from build123d import *

# Parameters (mm, degrees)
CROQUIS1_R                 = 1.35255
CROQUIS1_R_2               = 1.778
SALIENTE_EXTRUIR1_DEPTH    = 3.175
CROQUIS5_R                 = 2.55
CORTAR_EXTRUIR1_DEPTH      = 53.649355209
CORTAR_EXTRUIR2_DEPTH      = 53.649355209
CORTAR_EXTRUIR2_DEPTH_BACK = 53.649355209
CROQUIS10_R                = 2.078
CROQUIS10_R_2              = 1.65255
CROQUIS10_R_3              = 2.85
CORTAR_EXTRUIR3_DEPTH      = 53.649355209


with BuildPart() as part:
    # Croquis1 → Saliente-Extruir1 (new body)
    with BuildSketch(Plane.XZ):
        with BuildLine():
            Line((-6.02234, -19.2405), (-6.02234, -20.828))
            ThreePointArc((-6.02234, -20.828), (-5.836352806, -21.277012806), (-5.38734, -21.463))
            Line((-5.38734, -21.463), (0.96266, -21.463))
            ThreePointArc((0.96266, -21.463), (1.411672806, -21.277012806), (1.59766, -20.828))
            Line((1.59766, -20.828), (1.59766, -19.2405))
            ThreePointArc((1.59766, -19.2405), (2.062627985, -18.117967985), (3.18516, -17.653))
            Line((3.18516, -17.653), (36.43122, -17.653))
            ThreePointArc((36.43122, -17.653), (41.454190356, -15.572417555), (43.534772801, -10.549447199))
            Line((43.534772801, -10.549447199), (43.534772801, 10.549447199))
            ThreePointArc((43.534772801, 10.549447199), (41.454190356, 15.572417555), (36.43122, 17.653))
            Line((36.43122, 17.653), (3.18516, 17.653))
            ThreePointArc((3.18516, 17.653), (2.062627985, 18.117967985), (1.59766, 19.2405))
            Line((1.59766, 19.2405), (1.59766, 20.828))
            ThreePointArc((1.59766, 20.828), (1.411672806, 21.277012806), (0.96266, 21.463))
            Line((0.96266, 21.463), (-5.38734, 21.463))
            ThreePointArc((-5.38734, 21.463), (-5.836352806, 21.277012806), (-6.02234, 20.828))
            Line((-6.02234, 20.828), (-6.02234, 19.2405))
            ThreePointArc((-6.02234, 19.2405), (-6.487307985, 18.117967985), (-7.60984, 17.653))
            Line((-7.60984, 17.653), (-23.755604, 17.653))
            ThreePointArc((-23.755604, 17.653), (-24.878136015, 18.117967985), (-25.343104, 19.2405))
            Line((-25.343104, 19.2405), (-25.343104, 20.828))
            ThreePointArc((-25.343104, 20.828), (-25.529091194, 21.277012806), (-25.978104, 21.463))
            Line((-25.978104, 21.463), (-32.328104, 21.463))
            ThreePointArc((-32.328104, 21.463), (-32.777116806, 21.277012806), (-32.963104, 20.828))
            Line((-32.963104, 20.828), (-32.963104, 19.2405))
            ThreePointArc((-32.963104, 19.2405), (-33.428071985, 18.117967985), (-34.550604, 17.653))
            Line((-34.550604, 17.653), (-36.43122, 17.653))
            ThreePointArc((-36.43122, 17.653), (-44.591052878, 14.273086555), (-47.970966323, 6.113253677))
            Line((-47.970966323, 6.113253677), (-47.970966323, -6.113253677))
            ThreePointArc((-47.970966323, -6.113253677), (-44.591052878, -14.273086555), (-36.43122, -17.653))
            Line((-36.43122, -17.653), (-34.550604, -17.653))
            ThreePointArc((-34.550604, -17.653), (-33.428071985, -18.117967985), (-32.963104, -19.2405))
            Line((-32.963104, -19.2405), (-32.963104, -20.828))
            ThreePointArc((-32.963104, -20.828), (-32.777116806, -21.277012806), (-32.328104, -21.463))
            Line((-32.328104, -21.463), (-25.978104, -21.463))
            ThreePointArc((-25.978104, -21.463), (-25.529091194, -21.277012806), (-25.343104, -20.828))
            Line((-25.343104, -20.828), (-25.343104, -19.2405))
            ThreePointArc((-25.343104, -19.2405), (-24.878136015, -18.117967985), (-23.755604, -17.653))
            Line((-23.755604, -17.653), (-7.60984, -17.653))
            ThreePointArc((-7.60984, -17.653), (-6.487307985, -18.117967985), (-6.02234, -19.2405))
        make_face()
        with Locations(Location((33.655, -7.874, 0), (0, 0, 90))):
            Circle(CROQUIS1_R, mode=Mode.SUBTRACT)
        with Locations(Location((-33.655, 7.874, 0), (0, 0, 90))):
            Circle(CROQUIS1_R, mode=Mode.SUBTRACT)
        with Locations(Location((-33.655, -7.874, 0), (0, 0, 90))):
            Circle(CROQUIS1_R, mode=Mode.SUBTRACT)
        with Locations(Location((-2.21234, 18.288, 0), (0, 0, 90))):
            Circle(CROQUIS1_R_2, mode=Mode.SUBTRACT)
        with Locations(Location((-29.153104, -18.288, 0), (0, 0, 90))):
            Circle(CROQUIS1_R_2, mode=Mode.SUBTRACT)
        with Locations(Location((-2.21234, -18.288, 0), (0, 0, 90))):
            Circle(CROQUIS1_R_2, mode=Mode.SUBTRACT)
        with Locations(Location((-29.153104, 18.288, 0), (0, 0, 90))):
            Circle(CROQUIS1_R_2, mode=Mode.SUBTRACT)
        with Locations(Location((33.655, 7.874, 0), (0, 0, 90))):
            Circle(CROQUIS1_R, mode=Mode.SUBTRACT)
        with BuildLine():
            Line((-33.9725, 2.4765), (-30.827491336, 2.4765))
            Line((-30.827491336, 2.4765), (-30.827491336, 10.246241112))
            ThreePointArc((-30.827491336, 10.246241112), (-32.595430826, 12.971859774), (-30.143156557, 15.102812154))
            Line((-30.143156557, 15.102812154), (30.102172211, 15.102812154))
            ThreePointArc((30.102172211, 15.102812154), (32.54999843, 13.002076782), (30.845, 10.263843291))
            Line((30.845, 10.263843291), (30.845, 2.4765))
            Line((30.845, 2.4765), (33.9725, 2.4765))
            ThreePointArc((33.9725, 2.4765), (36.449, 0), (33.9725, -2.4765))
            Line((33.9725, -2.4765), (30.845, -2.4765))
            Line((30.845, -2.4765), (30.845, -10.263843291))
            ThreePointArc((30.845, -10.263843291), (32.539365892, -13.004061323), (30.092328369, -15.099694402))
            Line((30.092328369, -15.099694402), (-30.132404788, -15.099694402))
            ThreePointArc((-30.132404788, -15.099694402), (-32.583891793, -12.974283727), (-30.827491336, -10.246241112))
            Line((-30.827491336, -10.246241112), (-30.827491336, -2.4765))
            Line((-30.827491336, -2.4765), (-33.9725, -2.4765))
            ThreePointArc((-33.9725, -2.4765), (-36.449, 0), (-33.9725, 2.4765))
        make_face(mode=Mode.SUBTRACT)
    extrude(amount=-SALIENTE_EXTRUIR1_DEPTH)

    # Croquis5 → Cortar-Extruir1 (cut, through all)
    with BuildSketch(Plane(origin=(0, 3.175, 0), x_dir=(1, 0, 0), z_dir=(0, 1, 0))):
        with Locations(Location((-42.138904379, 0, 0), (0, 0, 270))):
            Circle(CROQUIS5_R)
    extrude(amount=-CORTAR_EXTRUIR1_DEPTH, mode=Mode.SUBTRACT)

    # Croquis9 → Cortar-Extruir2 (cut, two sides: drawn at the far end of the back side and taken through both)
    with BuildSketch(Plane(origin=(0, 3.175, 0), x_dir=(1, 0, 0), z_dir=(0, 1, 0)).offset(-CORTAR_EXTRUIR2_DEPTH_BACK)):
        with BuildLine():
            Line((30.845, -2.4765), (30.845, -3.75))
            Line((30.845, -3.75), (36.645, -3.75))
            ThreePointArc((36.645, -3.75), (40.395, 0), (36.645, 3.75))
            Line((36.645, 3.75), (30.845, 3.75))
            Line((30.845, 3.75), (30.845, 2.4765))
            Line((30.845, 2.4765), (33.9725, 2.4765))
            ThreePointArc((33.9725, 2.4765), (36.449, 0), (33.9725, -2.4765))
            Line((33.9725, -2.4765), (30.845, -2.4765))
        make_face()
    extrude(amount=CORTAR_EXTRUIR2_DEPTH + CORTAR_EXTRUIR2_DEPTH_BACK, mode=Mode.SUBTRACT)

    # Croquis10 → Cortar-Extruir3 (cut, through all)
    with BuildSketch(Plane(origin=(0, 3.175, 0), x_dir=(1, 0, 0), z_dir=(0, 1, 0))):
        with Locations(Location((-29.153104, 18.288, 0), (0, 0, 270))):
            Circle(CROQUIS10_R)
        with Locations(Location((-33.655, 7.874, 0), (0, 0, 270))):
            Circle(CROQUIS10_R_2)
        with Locations(Location((-42.138904379, 0, 0), (0, 0, 270))):
            Circle(CROQUIS10_R_3)
        with Locations(Location((-33.655, -7.874, 0), (0, 0, 270))):
            Circle(CROQUIS10_R_2)
        with Locations(Location((-29.153104, -18.288, 0), (0, 0, 270))):
            Circle(CROQUIS10_R)
        with Locations(Location((-2.21234, -18.288, 0), (0, 0, 270))):
            Circle(CROQUIS10_R)
        with Locations(Location((-2.21234, 18.288, 0), (0, 0, 270))):
            Circle(CROQUIS10_R)
        with Locations(Location((33.655, 7.874, 0), (0, 0, 270))):
            Circle(CROQUIS10_R_2)
        with Locations(Location((33.655, -7.874, 0), (0, 0, 270))):
            Circle(CROQUIS10_R_2)
    extrude(amount=-CORTAR_EXTRUIR3_DEPTH, mode=Mode.SUBTRACT)


solid = part.part
CAD build for the part. Positions are in the model's coordinates, mm. A direction names the side the tool comes from. Give positions to 0.01 mm unless a question says otherwise; leave off trailing zeros. Write each loop counter-clockwise with the first axis right and the second up, starting at its lowest first coordinate (ties: lowest second). Pieces come first, ordered by that corner, then holes. Notation, with made-up numbers: (12.25, 57.5) -> (36.25, 57.5) arc R15 ccw to (36.25, 80.5) -> close; hole circle Ø7 at (26.25, 15.5). An arc over 180 degrees is marked (long way). Return JSON: item names as keys, results as strings.
Item 1: Drill centre lines: probe 1 along Z at (x, y) = (-22.5, 2.5); probe 2 along X at (y, z) = (0.65, -4) (1 decimal); probe 3 along Z at (x, y) = (34, 1.6). Where is each one in solid material? Low to high.
Answer below:
{"probe 1": "z = -17.65 to -15.1, 15.1 to 17.65", "probe 2": "x = -48 to -30.8, 30.8 to 43.5", "probe 3": "z = -17.65 to -9.49, -6.26 to -3.75, 3.75 to 6.26, 9.49 to 17.65"}
Item 2: Band-saw the part on A-A (z = 0). List the corners of the cut face in (x, y) (3 decimals), then the cut area to 3 significant figures.
Answer below:
{"outline": "(-47.971, 0) -> (-44.989, 0) -> (-44.989, 3.175) -> (-47.971, 3.175) -> close; (-39.289, 0) -> (-36.449, 0) -> (-36.449, 3.175) -> (-39.289, 3.175) -> close; (40.395, 0) -> (43.535, 0) -> (43.535, 3.175) -> (40.395, 3.175) -> close", "area": "28.5 mm2"}
Item 3: Two-plate mould, pull along X, no slides. Class faces 4 (the flat face through (20, 2, -17.653)), 5 (the flat face through (-47.971, 2, 0)), 6 (the flat face through (-6.022, 2, 20)): +X half, -X half, draft (parallel to the pull), parting line (faces both ways), or undercut.
Answer below:
{"face 4": "draft", "face 5": "-X half", "face 6": "undercut"}
Item 4: Tool access for faces 1 (the flat face through (-32.963, 2, 20)), 2 (the cylindrical face through (32.542, 1.565, 13.051)), 3 (the cylindrical face through (-6.5, 1.565, -18.106)): list every direction of +Z, -Z, +X, -X, +Y, -Y with a clear straight run to the whole face (end or side of a thin tool).
Answer below:
{"face 1": "+Z, -X, +Y, -Y", "face 2": "+Y, -Y", "face 3": "-Z, +Y, -Y"}
Item 5: Band-saw the part on B-B (x = -12.5). List the corners of the cut face in (y, z) (3 decimals), then the cut area to 3 significant figures.
Answer below:
{"outline": "(0, -17.653) -> (3.175, -17.653) -> (3.175, -15.1) -> (0, -15.1) -> close; (0, 15.103) -> (3.175, 15.103) -> (3.175, 17.653) -> (0, 17.653) -> close", "area": "16.2 mm2"}
Item 6: Band-saw the part on D-D (y = 1.7). Give the number of separate pieces and of enclosed holes in the cut face, then the cut area to 3 significant figures.
Answer below:
{"separate pieces": "1", "enclosed holes": "10", "area": "1,180 mm2"}
Item 7: Drop flat-ended pins along their axis: pin 1 (1.7 mm diameter, centred on y = 2, z = 20, fed in from +X); pin 2 (2 mm diameter, centred on x = 33.655, z = -7.874, fed in from -Y); pin 3 (1.5 mm diameter, centred on x = -35.5, y = 2, fed in from +Z); pin 4 (1.7 mm diameter, centred on y = 2, z = -20, fed in from -X). Give the stop position or say it passes through.
Answer below:
{"pin 1": "stops at x = 1.6", "pin 2": "passes through", "pin 3": "stops at z = 17.65", "pin 4": "stops at x = -32.97"}
Item 8: Band-saw the part on C-C (z = -13.5). List the corners of the cut face in (x, y) (1 decimal), then the cut area to 3 significant figures.
Answer below:
{"outline": "(-45.3, 0) -> (-32.4, 0) -> (-32.4, 3.2) -> (-45.3, 3.2) -> close; (32.4, 0) -> (42.9, 0) -> (42.9, 3.2) -> (32.4, 3.2) -> close", "area": "74.1 mm2"}
